Read the model definition and answer for the solid it produces. Units are mm, in the model's axes. Face numbers are marked on the shaded views. A direction names the side the tool comes from. Coordinates: 2 decimals unless noted, no trailing zeros. Write each loop counter-clockwise with the first axis right and the second up, starting at its lowest first coordinate (ties: lowest second). Pieces come first, ordered by that corner, then holes. Notation, with made-up numbers: (38, -1) - (77, -1) arc R28 cw to (77, 31) - close; hole circle Ø5 at (49.5, 10). An arc over 180 degrees is marked (long way). Return JSON: item names as keys, results as strings.
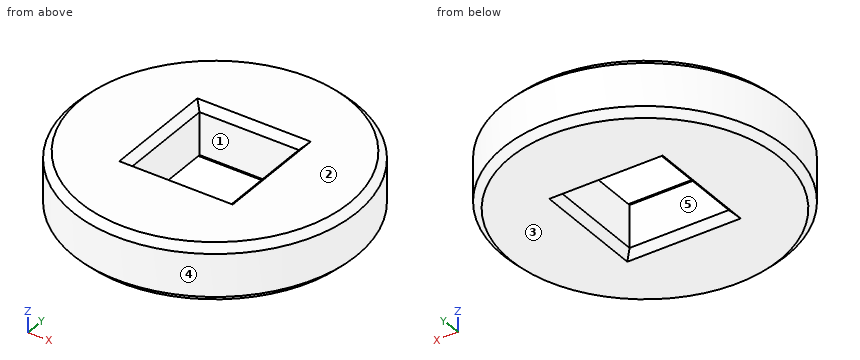
```python
from build123d import *

# Parameters (mm, degrees)
F0_R     = 10
F0_W     = 7
F0_H     = 7
F1_DEPTH = 4
F2_SIZE  = 0.5
F3_SIZE  = 0.5


with BuildPart() as f1:
    # F0 (on Top) → F1 (new body)
    with BuildSketch(Plane.XY):
        Circle(F0_R)
        Rectangle(F0_W, F0_H, mode=Mode.SUBTRACT)
    extrude(amount=F1_DEPTH)

    # F2
    f2_edges = [f1.edges().sort_by_distance(p)[0] for p in [
        (-10, 0, 4),
        (-10, 0, 0),
        (-3.5, 0, 0),
        (-3.5, 0, 4),
    ]]
    chamfer(f2_edges, length=F2_SIZE)

    # F3
    f3_edges = [f1.edges().sort_by_distance(p)[0] for p in [
        (0, 3.5, 4),
        (3.5, 0, 4),
        (0, -3.5, 4),
        (0, -3.5, 0),
        (0, 3.5, 0),
        (3.5, 0, 0),
        (-3.75, -3.5, 0),
        (-3.75, 3.5, 0),
        (-3.75, -3.5, 4),
        (-3.75, 3.5, 4),
    ]]
    chamfer(f3_edges, length=F3_SIZE)


solid = f1.part
```
(1) A cutting plane is placed at A-A (x = 0). Determine the outline of the cut face in (y, z), and give its area (3 significant figures).
Answer:
{"outline": "(-10, 0.5) - (-9.5, 0) - (-4, 0) - (-3.5, 0.5) - (-3.5, 3.5) - (-4, 4) - (-9.5, 4) - (-10, 3.5) - close; (3.5, 0.5) - (4, 0) - (9.5, 0) - (10, 0.5) - (10, 3.5) - (9.5, 4) - (4, 4) - (3.5, 3.5) - close", "area": "51.0 mm²"}
(2) Determine the mould class of the marked faces 3, 4 and 5 for opening direction X: +X half, -X half, draft (parallel to the pull), parting line (faces both ways), or undercut.
Answer:
{"face 3": "draft", "face 4": "parting line", "face 5": "undercut"}
(3) Straight lines are drawn through the part: line 1 (Y direction, x = 1, z = 1.25); line 2 (Y direction, x = -2.75, z = 1.65); line 3 (X direction, y = 0.5, z = 2.5). For each, find the intervals that lie inside material, in ascending order. Write a range as from..to.
Answer:
{"line 1": "-9.95..-3.5, 3.5..9.95", "line 2": "-9.61..-3.5, 3.5..9.61", "line 3": "-9.99..-3.5, 3.5..9.99"}
(4) A cutting plane is placed at C-C (z = 3.15). Determine the outline of the cut face in (x, y).
Answer:
{"outline": "circle Ø20 at (0, 0); hole (-3.5, -3.5) - (3.5, -3.5) - (3.5, 3.5) - (-3.5, 3.5) - close"}
(5) Which of the six approach directions +Z, -Z, +X, -X, +Y, -Y give full straight-line access (tool end or side, diameter ignored) to the marked faces 1 and 2?
Answer:
{"face 1": "+Z, -Z", "face 2": "+Z, +X, -X, +Y, -Y"}
(6) Flat-ended cylindrical pins translate along their axes: P1, Ø1, axis at y = 4, z = 2.5, coming from the +X side; P2, Ø1.5, axis at y = -1.5, z = 1.5, coming from the -X side; P3, Ø1.5, axis at x = 1, y = -1.5, coming from the +Z side. Find the tip coordinate at first contact, or state that the pin passes through.
Answer:
{"P1": "x = 9.37", "P2": "x = -9.97", "P3": "through"}
